Here's how the part is built. I have some questions about the finished solid (model axes, mm). Round coordinates to 2 decimals unless told otherwise and drop trailing zeros. Loops run counter-clockwise (first coordinate to the right, second up) from the corner with the lowest first, then second, coordinate; pieces in that order, holes last. Notation, with made-up numbers: M 48.25,2 L 90.25,2 A14 cw 90.25,16 Z; hole C -9,-20.75 d2. An arc over 180 degrees is marked long. Write item = value, one per line. Start each with the question number.
from build123d import *

# Parameters (mm, degrees)
SKIZZE1_R                       = 5
AUFSATZ_LINEAR_AUSTRAGEN1_DEPTH = 8.4


with BuildPart() as part:
    # Skizze1 → Aufsatz-Linear austragen1 (new body)
    with BuildSketch(Plane(origin=(0, 0, 0), x_dir=(1, 0, 0), z_dir=(0, 1, 0))):
        Polygon((0, 9.237604307), (-8, 4.618802154), (-8, -4.618802154), (0, -9.237604307), (8, -4.618802154), (8, 4.618802154), align=None)
        with Locations(Location((0, 0, 0), (0, 0, 270))):
            Circle(SKIZZE1_R, mode=Mode.SUBTRACT)
    extrude(amount=AUFSATZ_LINEAR_AUSTRAGEN1_DEPTH)

    # Skizze2 → Schnitt-Rotation1 (revolve, cut)
    with BuildSketch(Plane(origin=(0, 0, 0), x_dir=(0, 0, -1), z_dir=(1, 0, 0))):
        with BuildLine():
            Line((8.037604307, 8.4), (9.237604307, 8.4))
            Line((9.237604307, 8.4), (9.237604307, 7.9))
            ThreePointArc((9.237604307, 7.9), (8.687604307, 8.27), (8.037604307, 8.4))
        make_face()
        with BuildLine():
            Line((8.037604307, 0), (9.237604307, 0))
            Line((9.237604307, 0), (9.237604307, 0.5))
            ThreePointArc((9.237604307, 0.5), (8.687604307, 0.13), (8.037604307, 0))
        make_face()
    revolve(axis=Axis((0, 0, 0), (0, -1, 0)), mode=Mode.SUBTRACT)


solid = part.part
Item 1: Will these pins go through, and if not, where does the flat tip stop? pin 1 Ø2 at (x, y) = (2.5, 7) entering from +Z; pin 2 Ø1 at (x, y) = (4.5, 3.5) entering from -Z.
Item 2: I want a section at C-C, the plane x = -3.75. List the corners of the cut face in (y, z) for me, then the cut area to 3 significant figures.
Item 3: I want a section at A-A, the plane z = 0. List the corners of the cut face in (x, y) for me, then the cut area to 3 significant figures.
Item 4: I want a section at B-B, the plane y = 5.5. List the corners of the cut face in (x, z) for me.
Item 5: Please list where these lines run through material, in increasing order: line 1 (X direction, y = 5, z = 0); line 2 (Z direction, x = 3.25, y = 0.5); line 3 (X direction, y = 2.5, z = -1.5). Write a range as [from, to].
Item 6: We'd pull the mould along Z, two halves only. Please class faces 1 (the flat face through (8, 4, 0)), 2 (the flat face through (4.056, 4.141, -6.896)), 3 (the cylindrical face through (-4.88, 4.14, -1.08)): released by +Z, released by -Z, zero draft, split by the parting line, or undercut.
Worked out:
q1.pin_1 = 8.37
q1.pin_2 = -6.93
q2.outline = M 0,-7.07 L 8.4,-7.07 L 8.4,-3.31 L 0,-3.31 Z; M 0,3.31 L 8.4,3.31 L 8.4,7.07 L 0,7.07 Z
q2.area = 63.3 mm2
q3.outline = M -8,0 L -5,0 L -5,8.4 L -8,8.4 Z; M 5,0 L 8,0 L 8,8.4 L 5,8.4 Z
q3.area = 50.4 mm2
q4.outline = M -8,-4.62 L 0,-9.24 L 8,-4.62 L 8,4.62 L 0,9.24 L -8,4.62 Z; hole C 0,0 d10
q5.line_1 = [-8, -5], [5, 8]
q5.line_2 = [-7.36, -3.8], [3.8, 7.36]
q5.line_3 = [-8, -4.77], [4.77, 8]
q6.face_1 = zero draft
q6.face_2 = released by -Z
q6.face_3 = undercut
